Part model, mm, in its own coordinate system. Coordinates: 2 decimals unless noted, no trailing zeros. Order: outer loops, then holes, each group sorted by start corner. A loop starts at its lowest first (then second) coordinate and runs counter-clockwise, first axis right, second up.
from build123d import *

# Parameters (mm, degrees)
F0_W     = 152.4
F0_H     = 12.7
F0_R     = 3.1877
F1_DEPTH = 6.35
F3_D     = 2.7051
F4_D     = 2.7051
F5_D     = 2.7051


with BuildPart() as f1:
    # F0 (on Front) → F1 (new body)
    with BuildSketch(Plane.XZ):
        Rectangle(F0_W, F0_H)
        with Locations((-69.85, 1.27)):
            Circle(F0_R, mode=Mode.SUBTRACT)
        with Locations((69.85, 1.27)):
            Circle(F0_R, mode=Mode.SUBTRACT)
    extrude(amount=F1_DEPTH)

    # F3 (through all)
    with Locations(Plane(origin=(0, 0, -6.35), x_dir=(1, 0, 0), z_dir=(0, 0, -1))):
        with Locations((-57.15, 3.175), (57.15, 3.175)):
            Hole(F3_D / 2)

    # F4 (through all)
    with Locations(Plane(origin=(0, 0, -6.35), x_dir=(1, 0, 0), z_dir=(0, 0, -1))):
        with Locations((6.35, 3.175)):
            Hole(F4_D / 2)

    # F5 (through all)
    with Locations(Plane(origin=(0, 0, -6.35), x_dir=(1, 0, 0), z_dir=(0, 0, -1))):
        with Locations((38.1, 3.175)):
            Hole(F5_D / 2)


solid = f1.part
Q1. Cut at A-A on x = -57.15. Write the cut outline in (y, z), and give its area (3 significant figures).
Results list:
outline: (-6.35, -6.35) - (-4.53, -6.35) - (-4.53, 6.35) - (-6.35, 6.35) - close; (-1.82, -6.35) - (0, -6.35) - (0, 6.35) - (-1.82, 6.35) - close
area: 46.3 mm2
Q2. Cut at D-D on z = -5. Write the cut outline in (x, y) (3 decimals).
Results list:
outline: (-76.2, -6.35) - (76.2, -6.35) - (76.2, 0) - (-76.2, 0) - close; hole circle Ø2.705 at (-57.15, -3.175); hole circle Ø2.705 at (6.35, -3.175); hole circle Ø2.705 at (38.1, -3.175); hole circle Ø2.705 at (57.15, -3.175)
Q3. Wall check: line 1 along Y through (x, z) = (-57.15, -2); line 2 along X through (y, z) = (-5.5, 1.25); line 3 along X through (y, z) = (-4.75, 3). Give the ranges that are in metal, low to high.
Results list:
line 1: y = -6.35 to -4.53, -1.82 to 0
line 2: x = -76.2 to -73.04, -66.66 to 66.66, 73.04 to 76.2
line 3: x = -76.2 to -72.53, -67.17 to 67.17, 72.53 to 76.2
Q4. Cut at B-B on z = 1.27. Write the cut outline in (x, y) (3 decimals).
Results list:
outline: (-76.2, -6.35) - (-73.038, -6.35) - (-73.038, 0) - (-76.2, 0) - close; (-66.662, -6.35) - (66.662, -6.35) - (66.662, 0) - (-66.662, 0) - close; (73.038, -6.35) - (76.2, -6.35) - (76.2, 0) - (73.038, 0) - close; hole circle Ø2.705 at (-57.15, -3.175); hole circle Ø2.705 at (6.35, -3.175); hole circle Ø2.705 at (38.1, -3.175); hole circle Ø2.705 at (57.15, -3.175)
Q5. Pin check, flat tip, straight feed: pin 1 Ø2 at (x, y) = (-57.15, -3.175) entering from -Z. Stop position of the tip, or through.
Results list:
pin 1: passes through
Q6. Cut at C-C on x = 69.85. Write the cut outline in (y, z).
Results list:
outline: (-6.35, -6.35) - (0, -6.35) - (0, -1.92) - (-6.35, -1.92) - close; (-6.35, 4.46) - (0, 4.46) - (0, 6.35) - (-6.35, 6.35) - close
Q7. Mould opens along Z. For faces 1 (the face through (-73.035, -3.131, 1.41)), 2 (the face through (-1, 0, 0)), 3 (the face through (-1, -3, -6.35)) say: pulls with the +Z half, pulls with the -Z half, needs draft (parallel to the pull), parting line crosses it, or undercut.
Results list:
face 1: undercut
face 2: needs draft
face 3: pulls with the -Z half
